The model under review builds one solid part; all positions refer to its coordinate system, in mm. A direction names the side the tool comes from. Round coordinates to 2 decimals unless told otherwise and drop trailing zeros. Order: outer loops, then holes, each group sorted by start corner. A loop starts at its lowest first (then second) coordinate and runs counter-clockwise, first axis right, second up. Notation, with made-up numbers: M -13,68.25 L 11,68.25 A31 ccw 11,95.25 Z; hole C 21,-39 d6. An arc over 180 degrees is marked long. One line per item, written item: value. Start each with the question number.
Autodesk Inventor part; units mm, degrees
ref_plane "YZ Plane" through (0, 0, 0) normal (1, 0, 0) x (0, 1, 0)
ref_plane "XZ Plane" through (0, 0, 0) normal (0, 1, 0) x (-1, 0, 0)
ref_plane "XY Plane" through (0, 0, 0) normal (0, 0, 1) x (1, 0, 0)
sketch "Sketch1" plane through (0, 0, 0) normal (0, 0, 1) x (1, 0, 0)
  circle A0 centre (0, 0) radius 37.5
  dimension "d0" = 75
extrude "Extrusion1" add sketch "Sketch1" along normal mid plane 110
sketch "Sketch5" plane through (0, 0, 55) normal (0, 0, 1) x (1, 0, 0)
  circle A0 centre (0, 0) radius 39
  dimension "d22" = 78
extrude "Extrusion4" add sketch "Sketch5" against normal blind 4
mirror "Mirror2" about plane through (0, 0, 0) normal (0, 0, 1) of "Extrusion4"
sketch "Sketch4" plane through (0, 0, -55) normal (0, 0, -1) x (-1, 0, 0)
  point P0 (0, 0)
  point P1 (0, 0)
hole "Hole1" at (0, 0, -55) direction (0, 0, 1) diameter 26 end through all counterbore diameter 30.2 counterbore depth 9.3
mirror "Mirror1" about plane through (0, 0, 0) normal (0, 0, 1) of "Hole1"
properties part number "13042026-01"
Item 1: Consider section C-C, the plane z = -14.5. Give the boundary of the cut face in (x, y).
Item 2: Consider section D-D, the plane x = 18.5. Give the boundary of the cut face in (y, z).
Item 3: The part is to be moulded in two halves that separate along Z. For faces 1 (the flat face through (17, 1, 55)), 2 (the cylindrical face through (-4.88, 37.18, 0.71)), 3 (the cylindrical face through (-5.077, -38.668, -53.028)), say which applies: pulls with the +Z half, pulls with the -Z half, needs draft (parallel to the pull), parting line crosses it, or undercut.
Item 4: Wall thickness on L1, parallel to Y at x = 0, z = 49; L2, parallel to X at y = 6, z = -28.5: over which ranges is each line inside the solid? List them lowest first.
Item 5: Clearance check with flat-ended pins moving along their axes: P1, Ø5, axis at x = -20, z = -30, coming from the -Y side; P2, Ø5, axis at x = -5.5, z = -13.5, coming from the -Y side; P3, Ø10, axis at y = -11.5, z = 34.5, coming from the -X side; P4, Ø24, axis at x = 7, y = -5, coming from the +Z side. State where each tip first meets the part, or that it passes through.
Item 6: Consider section A-A, the plane x = 0. Give the boundary of the cut face in (y, z).
Item 7: Machinability: for faces 4 (the flat face through (-12.4, -4.4, 45.7)), 5 (the flat face through (-12.4, 4.4, -45.7)), 6 (the flat face through (-20, 32, 51)), which of the approach directions +Z, -Z, +X, -X, +Y, -Y give a long, thin tool a straight path to every point of the face, cutting with its end or side? Answer none if there is none.
Computed:
1. outline: C 0,0 d75; hole C 0,0 d26
2. outline: M -34.33,-55 L 34.33,-55 L 34.33,-51 L 32.62,-51 L 32.62,51 L 34.33,51 L 34.33,55 L -34.33,55 L -34.33,51 L -32.62,51 L -32.62,-51 L -34.33,-51 Z
3. face 1: pulls with the +Z half
3. face 2: undercut
3. face 3: needs draft
4. L1: y = -37.5 to -15.1, 15.1 to 37.5
4. L2: x = -37.02 to -11.53, 11.53 to 37.02
5. P1: stops at y = -33.17
5. P2: stops at y = -37.38
5. P3: stops at x = -36.93
5. P4: stops at z = 55
6. outline: M -39,-55 L -15.1,-55 L -15.1,-45.7 L -13,-45.7 L -13,45.7 L -15.1,45.7 L -15.1,55 L -39,55 L -39,51 L -37.5,51 L -37.5,-51 L -39,-51 Z; M 13,-45.7 L 15.1,-45.7 L 15.1,-55 L 39,-55 L 39,-51 L 37.5,-51 L 37.5,51 L 39,51 L 39,55 L 15.1,55 L 15.1,45.7 L 13,45.7 Z
7. face 4: +Z
7. face 5: -Z
7. face 6: none
